Geometry: final body of the model. Coordinates: model frame, mm. Coordinates: 2 decimals unless noted, no trailing zeros. Order: outer loops, then holes, each group sorted by start corner. A loop starts at its lowest first (then second) coordinate and runs counter-clockwise, first axis right, second up. Notation, with made-up numbers: M 9.25,-9.5 L 56.25,-9.5 A25 cw 56.25,28.5 Z; hole C 61.5,-37 d6. An arc over 180 degrees is marked long. Write item = value, one per line.
from build123d import *

# Parameters (mm, degrees)
SKETCH1_W           = 340
SKETCH1_H           = 165
BOSS_EXTRUDE1_DEPTH = 90
SKETCH2_R           = 5
BOSS_EXTRUDE2_DEPTH = 10


with BuildPart() as part:
    # Sketch1 → Boss-Extrude1 (new body)
    with BuildSketch(Plane(origin=(0, 0, 0), x_dir=(1, 0, 0), z_dir=(0, 1, 0))):
        Rectangle(SKETCH1_W, SKETCH1_H)
    extrude(amount=BOSS_EXTRUDE1_DEPTH)

    # Sketch2 → Boss-Extrude2 (add)
    with BuildSketch(Plane(origin=(0, 90, 0), x_dir=(1, 0, 0), z_dir=(0, 1, 0))):
        with Locations(Location((-165, -67.5, 0), (0, 0, 180))):
            Circle(SKETCH2_R)
        with Locations((165, -67.5)):
            Circle(SKETCH2_R)
    extrude(amount=BOSS_EXTRUDE2_DEPTH)


solid = part.part
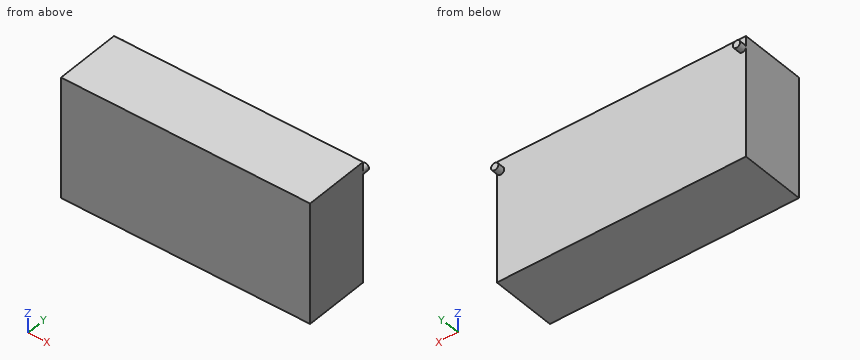
1) Section A-A, the plane x = -165. Return loops of the section in (y, z).
Numbers:
outline = M 0,-82.5 L 90,-82.5 L 90,62.5 L 100,62.5 L 100,72.5 L 90,72.5 L 90,82.5 L 0,82.5 Z
2) Section B-B, the plane z = -2.5. Return loops of the section in (x, y), and give its area (3 significant figures).
Numbers:
outline = M -170,0 L 170,0 L 170,90 L -170,90 Z
area = 30,600 mm²
3) Section C-C, the plane x = -46. Return loops of the section in (y, z), and give its area (4 significant figures).
Numbers:
outline = M 0,-82.5 L 90,-82.5 L 90,82.5 L 0,82.5 Z
area = 14,850 mm²
4) Line query: L1, parallel to Y at x = -150, z = 32. Output: solid intervals per line, ascending.
Numbers:
L1 = 0 to 90
